from build123d import *

# Parameters (mm, degrees)
BOSS_EXTRUDE1_DEPTH = 21
CUT_EXTRUDE1_START  = -5.9
CUT_EXTRUDE1_DEPTH  = 5.9
SKETCH3_W           = 10
SKETCH3_H           = 23.477945608
CUT_EXTRUDE2_DEPTH  = 0.5
CUT_EXTRUDE3_DEPTH  = 0.5
CUT_EXTRUDE4_DEPTH  = 11.5
BOSS_EXTRUDE2_DEPTH = 0.25
FILLET1_R           = 2.1
SKETCH7_R           = 2.5
BOSS_EXTRUDE3_DEPTH = 0.5
SKETCH8_W           = 0.5
SKETCH8_H           = 1.25
SKETCH8_H_2         = 0.5
SKETCH8_W_2         = 1.25
CUT_EXTRUDE5_DEPTH  = 0.1
FILLET2_R           = 2.49


# Read off the part's stored shape, not the designer's step: Cut-Extrude1
with BuildPart() as part:
    # Sketch1 → Boss-Extrude1 (new body)
    with BuildSketch(Plane.XY):
        with BuildLine():
            Line((0.012557203, -0.500251932), (-5.974554862, -0.89330298))
            Line((-5.974554862, -0.89330298), (-32.650528742, 3.842496807))
            ThreePointArc((-32.650528742, 3.842496807), (-35.431616847, 1.584631463), (-32.987442797, -1.0342271))
            Line((-32.987442797, -1.0342271), (0.012557203, -1.0342271))
            Line((0.012557203, -1.0342271), (0.012557203, -1.5342271))
            Line((0.012557203, -1.5342271), (-32.987442797, -1.5342271))
            ThreePointArc((-32.987442797, -1.5342271), (-35.930083434, 1.624018145), (-32.571991326, 4.336372166))
            Line((-32.571991326, 4.336372166), (-5.946831197, -0.390406628))
            Line((-5.946831197, -0.390406628), (0, 0))
            Line((0, 0), (0.012557203, -0.500251932))
        make_face()
    extrude(amount=BOSS_EXTRUDE1_DEPTH)

    # Cut-Extrude1 outline → Cut-Extrude1 (cut)
    with BuildSketch(Plane.XZ.offset(1.5342271).offset(CUT_EXTRUDE1_START)):
        with BuildLine():
            Line((0.012557203, 0), (0.012557203, 9.343939236))
            add(Edge.make_bspline(
                [(0.012557203, 9.343939236), (-0.067700916, 4.933400966), (-1.372327976, 0.5)],
                knots=[0.559253537, 0.559253537, 0.559253537, 1, 1, 1], degree=2))
            Line((-1.372327976, 0.5), (-5.946831197, 0.5))
            Line((-5.946831197, 0.5), (-32.987442797, 0))
            Line((-32.987442797, 0), (0.012557203, 0))
        make_face()
        with BuildLine():
            add(Edge.make_bspline(
                [(-1.755064488, 20.5), (-0.078758631, 15.514798295), (0.012557203, 10.5)],
                knots=[0, 0, 0, 0.501471147, 0.501471147, 0.501471147], degree=2))
            Line((0.012557203, 10.5), (0.012557203, 21))
            Line((0.012557203, 21), (-32.987442797, 21))
            Line((-32.987442797, 21), (-5.946831197, 20.5))
            Line((-5.946831197, 20.5), (-1.755064488, 20.5))
        make_face()
    extrude(amount=CUT_EXTRUDE1_DEPTH, mode=Mode.SUBTRACT)

    # Sketch3 → Cut-Extrude2 (cut)
    with BuildSketch(Plane.XZ.offset(1.5342271)):
        with Locations((-4.846794028, 9.392909882)):
            Rectangle(SKETCH3_W, SKETCH3_H)
    extrude(amount=-CUT_EXTRUDE2_DEPTH, mode=Mode.SUBTRACT)

    # Sketch4 → Cut-Extrude3 (cut)
    with BuildSketch(Plane.XZ.offset(1.5342271)):
        with BuildLine():
            Line((-22.987442797, 12), (-24.889366586, 12))
            ThreePointArc((-24.889366586, 12), (-30.487442797, 10.5), (-24.889366586, 9))
            Line((-24.889366586, 9), (-22.987442797, 9))
            ThreePointArc((-22.987442797, 9), (-21.487442797, 10.5), (-22.987442797, 12))
        make_face()
    extrude(amount=-CUT_EXTRUDE3_DEPTH, mode=Mode.SUBTRACT)

    # Sketch5 → Cut-Extrude4 (cut)
    with BuildSketch(Plane(origin=(0, -1.0342271, 0), x_dir=(1, 0, 0), z_dir=(0, 1, 0))):
        with BuildLine():
            Line((-27.487442797, -13.5), (-21.487442797, -13.5))
            ThreePointArc((-21.487442797, -13.5), (-18.487442797, -10.5), (-21.487442797, -7.5))
            Line((-21.487442797, -7.5), (-27.487442797, -7.5))
            ThreePointArc((-27.487442797, -7.5), (-30.487442797, -10.5), (-27.487442797, -13.5))
        make_face()
    extrude(amount=CUT_EXTRUDE4_DEPTH, mode=Mode.SUBTRACT)

    # Sketch6 → Boss-Extrude2 (add)
    with BuildSketch(Plane(origin=(-0.248891567, -1.401964872, 0), x_dir=(0.9846044320073983, -0.1747973468659884, 0), z_dir=(0.17479734686598838, 0.9846044320073982, 0))):
        with BuildLine():
            Line((-28.339083857, -3.5), (-15.339083857, -3.5))
            ThreePointArc((-15.339083857, -3.5), (-14.339083857, -4.5), (-15.339083857, -5.5))
            Line((-15.339083857, -5.5), (-28.339083857, -5.5))
            ThreePointArc((-28.339083857, -5.5), (-29.339083857, -4.5), (-28.339083857, -3.5))
        make_face()
        with BuildLine():
            Line((-28.339083857, -15.5), (-15.339083857, -15.5))
            ThreePointArc((-15.339083857, -15.5), (-14.339083857, -16.5), (-15.339083857, -17.5))
            Line((-15.339083857, -17.5), (-28.339083857, -17.5))
            ThreePointArc((-28.339083857, -17.5), (-29.339083857, -16.5), (-28.339083857, -15.5))
        make_face()
    extrude(amount=BOSS_EXTRUDE2_DEPTH)

    # Fillet1
    # the kernel refuses this fillet: 2.1 mm, written as the material it takes off along each edge
    with BuildSketch(Plane(origin=(-28.107979795, 3.797782907, 3.5), x_dir=(-0.1747973468659884, -0.9846044320073982, 0), z_dir=(0.9846044320073983, -0.1747973468659884, 0)), Plane(origin=(-15.308122178, 1.525417398, 5.5), x_dir=(-0.17479734686598844, -0.9846044320073983, 0), z_dir=(-0.9846044320073983, 0.1747973468659884, 0)), Plane(origin=(-28.107979795, 3.797782907, 15.5), x_dir=(-0.1747973468659884, -0.9846044320073983, 0), z_dir=(0.9846044320073983, -0.1747973468659884, 0)), Plane(origin=(-15.308122178, 1.525417398, 17.5), x_dir=(-0.17479734686598838, -0.9846044320073983, 0), z_dir=(-0.9846044320073983, 0.1747973468659884, 0))) as fillet1_piece_1:
        with BuildLine():
            CenterArc((2.1, -0.993730346), FILLET1_R, 151.757462816, 28.242537184)
            Line((0, -0.993730346), (-0.042, -0.993730346))
            Line((-0.042, -0.993730346), (-0.042, 0))
            Line((-0.042, 0), (0, 0.042))
            ThreePointArc((0, 0.042), (0.125, 0.042), (0.213, 0.019874607))
            Line((0.213, 0.019874607), (0.25, 0))
        make_face()
    extrude(amount=13, mode=Mode.SUBTRACT)
    with BuildSketch(Plane(origin=(-15.308122178, 1.525417398, 16.5), x_dir=(0, 0, -1), z_dir=(-0.9846044320073983, 0.1747973468659884, 0))) as fillet1_piece_2:
        with BuildLine():
            CenterArc((0.006269654, 2.1), FILLET1_R, 270, 28.242537184)
            Line((0.006269654, 0), (0.006269654, -0.042))
            Line((0.006269654, -0.042), (1, -0.042))
            Line((1, -0.042), (1.042, 0))
            ThreePointArc((1.042, 0), (1.042, 0.125), (1.019874607, 0.213))
            Line((1.019874607, 0.213), (1, 0.25))
        make_face()
    revolve(axis=Axis((-15.308122178, 1.525417398, 16.5), (-0.1747973468659884, -0.9846044320073983, 0)), revolution_arc=180, mode=Mode.SUBTRACT)
    with BuildSketch(Plane(origin=(-28.107979795, 3.797782907, 16.5), x_dir=(0, 0, 1), z_dir=(0.9846044320073983, -0.1747973468659884, 0))) as fillet1_piece_3:
        with BuildLine():
            CenterArc((0.006269654, 2.1), FILLET1_R, 270, 28.242537184)
            Line((0.006269654, 0), (0.006269654, -0.042))
            Line((0.006269654, -0.042), (1, -0.042))
            Line((1, -0.042), (1.042, 0))
            ThreePointArc((1.042, 0), (1.042, 0.125), (1.019874607, 0.213))
            Line((1.019874607, 0.213), (1, 0.25))
        make_face()
    revolve(axis=Axis((-28.107979795, 3.797782907, 16.5), (-0.1747973468659884, -0.9846044320073983, 0)), revolution_arc=180, mode=Mode.SUBTRACT)
    with BuildSketch(Plane(origin=(-15.308122178, 1.525417398, 4.5), x_dir=(0, 0, -1), z_dir=(-0.9846044320073983, 0.1747973468659884, 0))) as fillet1_piece_4:
        with BuildLine():
            CenterArc((0.006269654, 2.1), FILLET1_R, 270, 28.242537184)
            Line((0.006269654, 0), (0.006269654, -0.042))
            Line((0.006269654, -0.042), (1, -0.042))
            Line((1, -0.042), (1.042, 0))
            ThreePointArc((1.042, 0), (1.042, 0.125), (1.019874607, 0.213))
            Line((1.019874607, 0.213), (1, 0.25))
        make_face()
    revolve(axis=Axis((-15.308122178, 1.525417398, 4.5), (-0.1747973468659884, -0.9846044320073983, 0)), revolution_arc=180, mode=Mode.SUBTRACT)
    with BuildSketch(Plane(origin=(-28.107979795, 3.797782907, 4.5), x_dir=(0, 0, 1), z_dir=(0.9846044320073983, -0.1747973468659884, 0))) as fillet1_piece_5:
        with BuildLine():
            CenterArc((0.006269654, 2.1), FILLET1_R, 270, 28.242537184)
            Line((0.006269654, 0), (0.006269654, -0.042))
            Line((0.006269654, -0.042), (1, -0.042))
            Line((1, -0.042), (1.042, 0))
            ThreePointArc((1.042, 0), (1.042, 0.125), (1.019874607, 0.213))
            Line((1.019874607, 0.213), (1, 0.25))
        make_face()
    revolve(axis=Axis((-28.107979795, 3.797782907, 4.5), (-0.1747973468659884, -0.9846044320073983, 0)), revolution_arc=180, mode=Mode.SUBTRACT)

    # Sketch7 → Boss-Extrude3 (add)
    with BuildSketch(Plane(origin=(0, -1.0342271, 0), x_dir=(1, 0, 0), z_dir=(0, 1, 0))):
        with Locations(Location((-22.987442797, -10.5, 0), (0, 0, 218.942441269))):
            Circle(SKETCH7_R)
    extrude(amount=BOSS_EXTRUDE3_DEPTH)

    # Sketch8 → Cut-Extrude5 (cut)
    with BuildSketch(Plane(origin=(0, -0.5342271, 0), x_dir=(1, 0, 0), z_dir=(0, 1, 0))):
        with Locations((-22.987442797, -11.375)):
            Rectangle(SKETCH8_W, SKETCH8_H)
        with Locations((-22.987442797, -10.5)):
            Rectangle(SKETCH8_W, SKETCH8_H_2)
        with Locations((-22.987442797, -9.625)):
            Rectangle(SKETCH8_W, SKETCH8_H)
        with Locations((-23.862442797, -10.5)):
            Rectangle(SKETCH8_W_2, SKETCH8_H_2)
        with Locations((-22.112442797, -10.5)):
            Rectangle(SKETCH8_W_2, SKETCH8_H_2)
    extrude(amount=-CUT_EXTRUDE5_DEPTH, mode=Mode.SUBTRACT)

    # Fillet2
    # the kernel refuses this fillet: 2.49 mm, written as the material it takes off along each edge
    with BuildSketch(Plane(origin=(-22.987442797, -0.5342271, 10.5), x_dir=(-0.777777777777574, 0, 0.6285393610549612), z_dir=(-0.6285393610549612, 0, -0.777777777777574))) as fillet2_piece_1:
        with BuildLine():
            CenterArc((1.003337045, -2.49), FILLET2_R, 53.053469485, 36.946530515)
            Line((1.003337045, 0), (1.003337045, 0.0498))
            Line((1.003337045, 0.0498), (2.5, 0.0498))
            Line((2.5, 0.0498), (2.5498, 0))
            ThreePointArc((2.5498, 0), (2.5498, -0.25), (2.529933259, -0.4602))
            Line((2.529933259, -0.4602), (2.5, -0.5))
        make_face()
    revolve(axis=Axis((-22.987442797, -0.5342271, 10.5), (0, 1, 0)), mode=Mode.SUBTRACT)


solid = part.part
Source: CAD feature listing. Evaluate the final solid. Frame: model axes, mm. A direction names the side the tool comes from. Give positions to 0.01 mm unless a question says otherwise; leave off trailing zeros. Write each loop counter-clockwise with the first axis right and the second up, starting at its lowest first coordinate (ties: lowest second). Pieces come first, ordered by that corner, then holes. Notation, with made-up numbers: M 27,72.5 L 66,72.5 A6 cw 66,77.5 Z; hole C -28,18.25 d2. An arc over 180 degrees is marked long. Answer as a JSON object with one key per item and string values.
Q1. Ray query, line 1 along Y through (x, z) = (-17, 9.75); line 2 along X through (y, z) = (-1.3, 10.5); line 3 along Y through (x, z) = (-19.5, 19.25). Return the intervals inside material, ascending.
Geometry check:
{"line 1": "y = -1.53 to -1.03, 1.06 to 1.57", "line 2": "x = -34.14 to -30.49, -21.49 to -9.85", "line 3": "y = -1.53 to -1.03, 1.51 to 2.02"}
Q2. Mould query, pull axis Z, two halves, no side actions, for faces 6 (the face through (-2.939, -0.694, 10.36)), 7 (the face through (-21.63, 2.58, 17.03)), 8 (the face through (-30.487, 3.619, 10.434)). Classes: +Z half, -Z half, draft (parallel to the pull), parting line (faces both ways), or undercut.
Geometry check:
{"face 6": "draft", "face 7": "+Z half", "face 8": "undercut"}
Q3. Contact query for flat-ended pins moving along their axis: P1, Ø1.5, axis at x = -7, y = 0, coming from the +Z side; P2, Ø2, axis at x = -30.5, z = 10.5, coming from the +Y side; P3, Ø0.8, axis at x = -22.5, z = 10, coming from the +Y side. Output: stop coordinate, or through.
Geometry check:
{"P1": "stops at z = 20.53", "P2": "stops at y = 4.15", "P3": "stops at y = -0.53"}
Q4. Access query for faces 1 (the face through (-21.63, 2.58, 5.03)), 2 (the face through (-3.02, -0.2, 10.36)), 3 (the face through (-24, -1.034, 10)), 4 (the face through (-16.162, 0.915, 10.353)), 5 (the face through (-24.5, 2.6, 7.5)). Directions: +Z, -Z, +X, -X, +Y, -Y. A direction counts if a zero-diameter tool reaches every point of the face in a straight line with its end or side. Return the directions, or none.
Geometry check:
{"face 1": "+X, +Y", "face 2": "+Z, -Z, +Y", "face 3": "-Y", "face 4": "+Z, -Z", "face 5": "+Y"}
Q5. Cut plane B-B, the plane x = -20. Count the separate pieces of the cut face and the enclosed holes in it, then the cut area to 3 significant figures.
Geometry check:
{"separate pieces": "3", "enclosed holes": "0", "area": "18.7 mm^2"}
Q6. Cut plane A-A, the plane x = -12.5. Return the cut outline in (y, z), then the cut area to 3 significant figures.
Geometry check:
{"outline": "M -1.53,0.38 L -1.03,0.38 L -1.03,20.62 L -1.53,20.62 Z; M 0.27,0.38 L 0.77,0.38 L 0.77,20.62 L 0.27,20.62 Z", "area": "20.4 mm^2"}
